The model under review builds one solid part; all positions refer to its coordinate system, in mm. A direction names the side the tool comes from. Round coordinates to 2 decimals unless told otherwise and drop trailing zeros. Loops run counter-clockwise (first coordinate to the right, second up) from the corner with the lowest first, then second, coordinate; pieces in that order, holes last. Notation, with made-up numbers: (61.5, -7) - (92.5, -7) arc R22 ccw to (92.5, 17) - close; hole circle Ø9 at (-28.75, -33.75). An arc over 180 degrees is marked (long way). Answer as CSV lines item,"result".
from build123d import *

# Parameters (mm, degrees)
BOSS_EXTRUDE1_DEPTH = 150


with BuildPart() as part:
    # Sketch1 → Boss-Extrude1 (new body)
    with BuildSketch(Plane.XY):
        with BuildLine():
            Line((-17.933849058, 1.310471954), (-17.438874304, 1.805446694))
            ThreePointArc((-17.438874304, 1.805446694), (-17.351006338, 2.017578728), (-17.438874304, 2.229710762))
            Line((-17.438874304, 2.229710762), (-18.936235421, 3.72707188))
            ThreePointArc((-18.936235421, 3.72707188), (-19.116679575, 4.6342259), (-18.347631531, 5.148087374))
            Line((-18.347631531, 5.148087374), (-15.165219907, 5.148087374))
            ThreePointArc((-15.165219907, 5.148087374), (-14.01716961, 4.919725971), (-13.043899564, 4.269407717))
            Line((-13.043899564, 4.269407717), (-11.439379376, 2.66488753))
            ThreePointArc((-11.439379376, 2.66488753), (-10.789061123, 1.691617485), (-10.560699721, 0.54356719))
            Line((-10.560699721, 0.54356719), (-10.560699721, -2.638844434))
            ThreePointArc((-10.560699721, -2.638844434), (-11.074561199, -3.407892483), (-11.981715225, -3.227448328))
            Line((-11.981715225, -3.227448328), (-13.479076343, -1.730087211))
            ThreePointArc((-13.479076343, -1.730087211), (-13.691208377, -1.642219245), (-13.903340412, -1.730087211))
            Line((-13.903340412, -1.730087211), (-14.398315158, -2.225061958))
            ThreePointArc((-14.398315158, -2.225061958), (-14.632629733, -2.790747383), (-14.398315158, -3.356432808))
            Line((-14.398315158, -3.356432808), (-11.091426526, -6.66332144))
            Line((-11.091426526, -6.66332144), (-11.021736276, -6.72655883))
            ThreePointArc((-11.021736276, -6.72655883), (-9.637071865, -7.232037367), (-8.282153045, -6.651521154))
            ThreePointArc((-8.282153045, -6.651521154), (-0.986587883, 4.879678298), (2.008460712, 18.19221058))
            ThreePointArc((2.008460712, 18.19221058), (1.440783284, 19.581695132), (0.06638279, 20.184976381))
            ThreePointArc((0.06638279, 20.184976381), (0.035983891, 20.186304583), (0.00556439, 20.187019567))
            Line((0.00556439, 20.187019567), (-4.64176753, 20.187019567))
            ThreePointArc((-4.64176753, 20.187019567), (-5.207452955, 19.952704992), (-5.44176753, 19.387019567))
            Line((-5.44176753, 19.387019567), (-5.44176754, 18.687019567))
            ThreePointArc((-5.44176754, 18.687019567), (-5.353899574, 18.474887532), (-5.14176754, 18.387019567))
            Line((-5.14176754, 18.387019567), (-3.02417914, 18.387019567))
            ThreePointArc((-3.02417914, 18.387019567), (-2.255131096, 17.873158092), (-2.43557525, 16.966004073))
            Line((-2.43557525, 16.966004073), (-4.68588009, 14.715699233))
            ThreePointArc((-4.68588009, 14.715699233), (-5.659150136, 14.065380979), (-6.807200433, 13.837019576))
            Line((-6.807200433, 13.837019576), (-9.076334643, 13.837019576))
            ThreePointArc((-9.076334643, 13.837019576), (-10.224384938, 14.065380978), (-11.197654983, 14.715699231))
            Line((-11.197654983, 14.715699231), (-13.447959823, 16.966004071))
            ThreePointArc((-13.447959823, 16.966004071), (-13.628403978, 17.873158097), (-12.859355929, 18.387019575))
            Line((-12.859355929, 18.387019575), (-10.741767529, 18.387019575))
            ThreePointArc((-10.741767529, 18.387019575), (-10.529635495, 18.474887541), (-10.441767529, 18.687019575))
            Line((-10.441767529, 18.687019575), (-10.441767529, 19.387019575))
            ThreePointArc((-10.441767529, 19.387019575), (-10.676082104, 19.952705), (-11.241767529, 20.187019575))
            Line((-11.241767529, 20.187019575), (-16.032865229, 20.187019575))
            ThreePointArc((-16.032865229, 20.187019575), (-17.381264954, 19.664117467), (-18.02458362, 18.368837756))
            ThreePointArc((-18.02458362, 18.368837756), (-19.464176878, 12.533350929), (-22.57254303, 7.389092466))
            ThreePointArc((-22.57254303, 7.389092466), (-23.035584519, 6.097289793), (-22.557062201, 4.811141295))
            Line((-22.557062201, 4.811141295), (-22.41767475, 4.662926796))
            Line((-22.41767475, 4.662926796), (-19.065219908, 1.310471954))
            ThreePointArc((-19.065219908, 1.310471954), (-18.499534483, 1.076157379), (-17.933849058, 1.310471954))
        make_face()
        with BuildLine():
            Line((-12.14365631, 13.117817809), (-15.63660261, 16.610764109))
            ThreePointArc((-15.63660261, 16.610764109), (-16.139874769, 16.734268673), (-16.482327269, 16.345343836))
            ThreePointArc((-16.482327269, 16.345343836), (-17.800420542, 11.845449218), (-20.050293851, 7.731510528))
            ThreePointArc((-20.050293851, 7.731510528), (-20.083154751, 7.214348654), (-19.63995668, 6.945812413))
            Line((-19.63995668, 6.945812413), (-14.70018465, 6.945812413))
            ThreePointArc((-14.70018465, 6.945812413), (-14.301543386, 7.144009261), (-14.21893989, 7.581471843))
            ThreePointArc((-14.21893989, 7.581471843), (-14.058708433, 10.295581323), (-12.252843967, 12.328047292))
            ThreePointArc((-12.252843967, 12.328047292), (-12.001920705, 12.695789539), (-12.14365631, 13.117817809))
        make_face(mode=Mode.SUBTRACT)
        with BuildLine():
            Line((-0.870882283, 15.9852679), (-6.207568998, 10.648581185))
            ThreePointArc((-6.207568998, 10.648581185), (-6.342128781, 10.40340459), (-6.323971818, 10.124319975))
            ThreePointArc((-6.323971818, 10.124319975), (-6.390508312, 7.119308828), (-8.468323669, 4.947396666))
            ThreePointArc((-8.468323669, 4.947396666), (-8.678505203, 4.762892953), (-8.7567231, 4.494378786))
            Line((-8.7567231, 4.494378786), (-8.7567231, -3.052835944))
            ThreePointArc((-8.7567231, -3.052835944), (-8.419748711, -3.525511996), (-7.8630325, -3.361069154))
            ThreePointArc((-7.8630325, -3.361069154), (-2.648796205, 5.569440932), (-0.020993808, 15.571287015))
            ThreePointArc((-0.020993808, 15.571287015), (-0.298372973, 16.081223462), (-0.870882283, 15.9852679))
        make_face(mode=Mode.SUBTRACT)
        with BuildLine():
            ThreePointArc((-12.37538155, 8.706516606), (-10.22538155, 6.556516606), (-8.07538155, 8.706516606))
            ThreePointArc((-8.07538155, 8.706516606), (-10.22538155, 10.856516606), (-12.37538155, 8.706516606))
        make_face(mode=Mode.SUBTRACT)
    extrude(amount=BOSS_EXTRUDE1_DEPTH)


solid = part.part
1. Wall thickness on probe 1 along X at (y, z) = (12.5, 133); probe 2 along X at (y, z) = (15.5, 35.5); probe 3 along Y at (x, z) = (-2.5, 52.5): over which ranges is each line inside the solid? List them lowest first.
Numbers:
probe 1,"x = -19.48 to -17.54, -12.07 to -4.36, -0.52 to 1.31"
probe 2,"x = -18.5 to -16.65, -14.53 to -11.98, -3.9 to -1.36, -0.03 to 1.78"
probe 3,"y = 1.64 to 5.93, 14.36 to 16.9, 18.2 to 20.19"
2. Take a section at A-A (y = -5). State the section outline as (x, z) points, plus the area to 3 significant figures.
Numbers:
outline,"(-12.75, 0) - (-6.87, 0) - (-6.87, 150) - (-12.75, 150) - close"
area,"883 mm²"
3. Clearance check with flat-ended pins moving along their axes: pin 1 (0.6 mm diameter, centred on x = -11.5, z = 66.5, fed in from -Y); pin 2 (2.5 mm diameter, centred on x = -18, z = 42, fed in from +Y); pin 3 (4 mm diameter, centred on y = 2.5, z = 54, fed in from +X). State where each tip first meets the part, or that it passes through.
Numbers:
pin 1,"stops at y = -6.55"
pin 2,"stops at y = 20.05"
pin 3,"stops at x = -1.15"
4. Take a section at B-B (z = 103.5). State how many separate pieces and enclosed holes the cut face has, plus the area to 3 significant figures.
Numbers:
separate pieces,"1"
enclosed holes,"3"
area,"239 mm²"
5. Draft analysis for pull direction Y (two halves, no side actions). For faces 1 (the face through (-12.768, -4.987, 73.95)), 2 (the face through (-3.502, 13.354, 73.95)), 3 (the face through (-8, 10, 150)), state which applies: +Y half, -Y half, draft (parallel to the pull), parting line (faces both ways), or undercut.
Numbers:
face 1,"-Y half"
face 2,"undercut"
face 3,"draft"
6. Tool access review of faces 4 (the face through (-8, 10, 0)), 5 (the face through (-13.866, 14.84, 73.95)): name each direction out of +Z, -Z, +X, -X, +Y, -Y from which nothing blocks a thin tool from reaching the whole face with its end or side.
Numbers:
face 4,"-Z, +X, -X, +Y, -Y"
face 5,"+Z, -Z"
